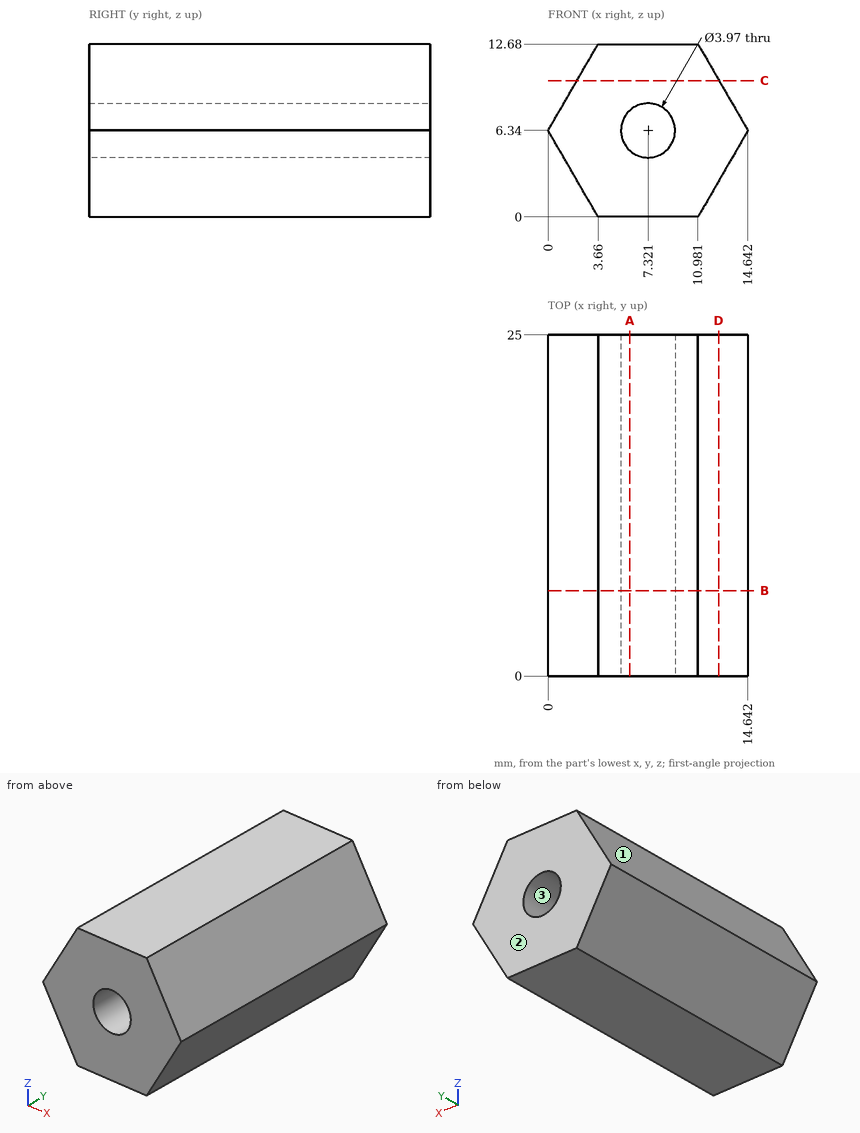
The figure shows three views and two pictorial views of one solid part (mm, origin at its lowest corner). Answer the questions. Round coordinates to 2 decimals unless told otherwise and drop trailing zeros. Write each loop counter-clockwise with the first axis right and the second up, starting at its lowest first coordinate (ties: lowest second). Pieces come first, ordered by that corner, then holes. Notation, with made-up numbers: M -27,-19.75 L -20,-19.75 A21 cw -20,-3.75 Z; hole C 84.25,78 d4. An arc over 180 degrees is marked long. Use a Markdown table: item, result.
1) The part is cut by section D-D on x = 12.5. Give the vertices of the cut face in (y, z).
Taken from the geometry:
| item | result |
|---|---|
| outline | M 0,2.63 L 25,2.63 L 25,10.05 L 0,10.05 Z |
2) The part is cut by section B-B on y = 6.25. Give the vertices of the cut face in (x, z) (1 decimal).
Taken from the geometry:
| item | result |
|---|---|
| outline | M 0,6.3 L 3.7,0 L 11,0 L 14.6,6.3 L 11,12.7 L 3.7,12.7 Z; hole C 7.3,6.3 d4 |
3) Consider line 1 (Z direction, x = 9, y = 23.5); line 2 (Z direction, x = 7.75, y = 10.5); line 3 (X direction, y = 20.25, z = 5) (1 decimal). Determine where each line is inside the solid, lowest interval first. Write a range as [from, to].
Taken from the geometry:
| item | result |
|---|---|
| line 1 | z = [0, 5.28], [7.4, 12.68] |
| line 2 | z = [0, 4.4], [8.28, 12.68] |
| line 3 | x = [0.8, 5.9], [8.8, 13.9] |
4) Flat-ended cylindrical pins translate along their axes: pin 1 (1 mm diameter, centred on y = 14.5, z = 2.5, fed in from +X); pin 2 (4 mm diameter, centred on y = 8, z = 3.5, fed in from +X); pin 3 (1 mm diameter, centred on y = 10.5, z = 1.5, fed in from +X) (1 decimal). Find the tip coordinate at first contact, or state that the pin passes through.
Taken from the geometry:
| item | result |
|---|---|
| pin 1 | stops at x = 12.71 |
| pin 2 | stops at x = 14.16 |
| pin 3 | stops at x = 12.1 |
5) The part is cut by section A-A on x = 6. Give the vertices of the cut face in (y, z), plus the area to 3 significant figures.
Taken from the geometry:
| item | result |
|---|---|
| outline | M 0,0 L 25,0 L 25,4.86 L 0,4.86 Z; M 0,7.82 L 25,7.82 L 25,12.68 L 0,12.68 Z |
| area | 243 mm2 |
6) Determine the mould class of the marked faces 1, 2 and 3 for opening direction X: pulls with the +X half, pulls with the -X half, needs draft (parallel to the pull), parting line crosses it, or undercut.
Taken from the geometry:
| item | result |
|---|---|
| face 1 | pulls with the -X half |
| face 2 | needs draft |
| face 3 | undercut |
7) The part is cut by section C-C on z = 10. Give the vertices of the cut face in (x, y), plus the area to 3 significant figures.
Taken from the geometry:
| item | result |
|---|---|
| outline | M 2.11,0 L 12.53,0 L 12.53,25 L 2.11,25 Z |
| area | 260 mm2 |
